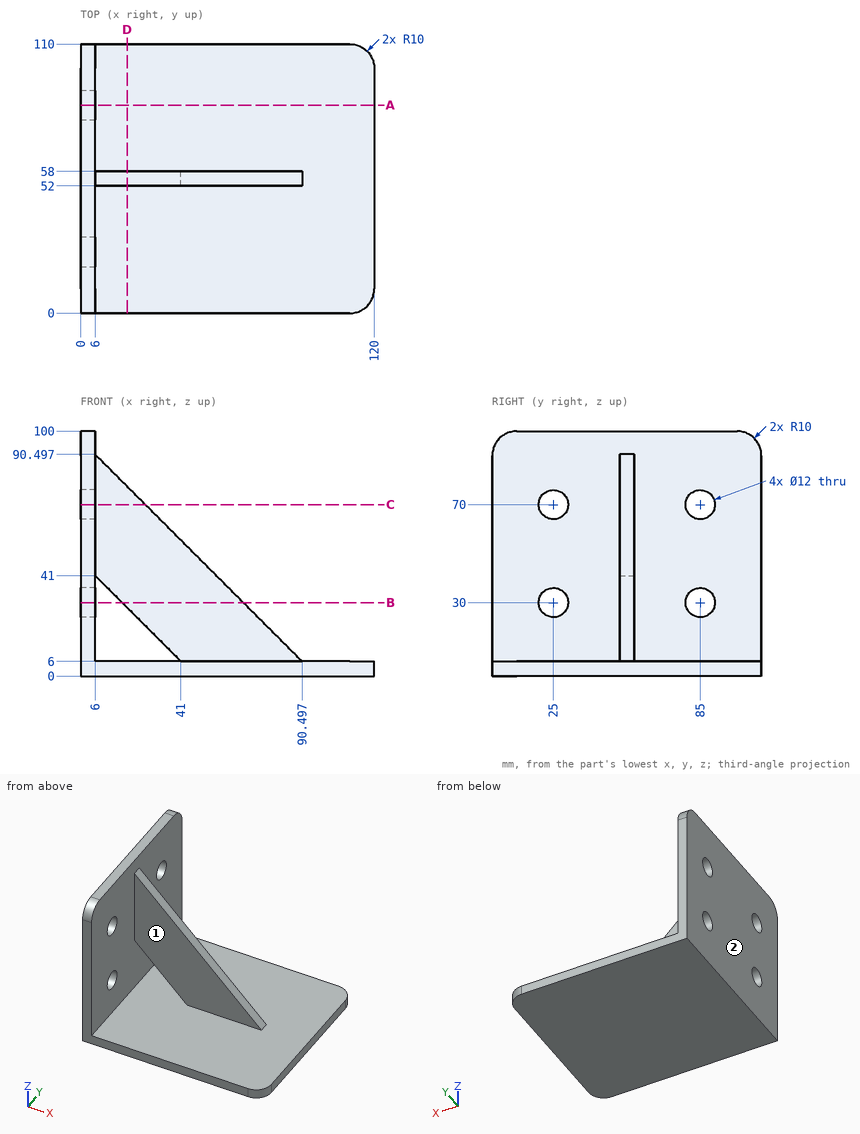
Verification items for this drawing (mm, ordinates from the low corner). Coordinates: 2 decimals unless noted, no trailing zeros. Order: outer loops, then holes, each group sorted by start corner. A loop starts at its lowest first (then second) coordinate and runs counter-clockwise, first axis right, second up. Notation, with made-up numbers: (25, 16.5) - (34, 16.5) arc R19 cw to (34, 29.5) - close; hole circle Ø9 at (-10.75, 4.5). An arc over 180 degrees is marked (long way). Answer as a JSON object with one key per item and string values. Group by question number.
Item 1: Sectioned sample at C-C, the plane z = 70. Record the cut outline in (x, y).
Item 2: Sectioned sample at D-D, the plane x = 19. Record the cut outline in (y, z), and give its area (3 significant figures).
Item 3: Depth check by flat-ended pin: pin 1 Ø11 at (y, z) = (25, 30) entering from +X; pin 2 Ø1 at (x, y) = (93, 98) entering from +Z; pin 3 Ø12 at (x, z) = (17, 32.5) entering from +Y. Enter the tip coordinate at first touch or a pass-through.
Item 4: Sectioned sample at B-B, the plane z = 30. Record the cut outline in (x, y).
Item 5: Draft check along X on the marked faces 1 and 2. Enter one of: +X half, -X half, draft (parallel to the pull), parting line (faces both ways), or undercut.
Item 6: Sectioned sample at A-A, the plane y = 85. Record the cut outline in (x, z).
Item 7: Scan lines: probe 1 along Z at (x, y) = (2.95, 85); probe 2 along X at (y, z) = (67.5, 87.5); probe 3 along Y at (x, z) = (9, 57.5). Record each from-to range of solid material in increasing order.
Resolved:
{
 "1": {"outline": "(0, 0) - (6, 0) - (6, 19) - (0, 19) - close; (0, 31) - (6, 31) - (6, 52) - (26.5, 52) - (26.5, 58) - (6, 58) - (6, 79) - (0, 79) - close; (0, 91) - (6, 91) - (6, 110) - (0, 110) - close"},
 "2": {"outline": "(0, 0) - (110, 0) - (110, 6) - (0, 6) - close; (52, 28) - (58, 28) - (58, 77.5) - (52, 77.5) - close", "area": "957 mm^2"},
 "3": {"pin 1": "through", "pin 2": "z = 6", "pin 3": "y = 58"},
 "4": {"outline": "(0, 0) - (6, 0) - (6, 19) - (0, 19) - close; (0, 31) - (6, 31) - (6, 79) - (0, 79) - close; (0, 91) - (6, 91) - (6, 110) - (0, 110) - close; (17, 52) - (66.5, 52) - (66.5, 58) - (17, 58) - close"},
 "5": {"face 1": "draft", "face 2": "-X half"},
 "6": {"outline": "(0, 0) - (120, 0) - (120, 6) - (6, 6) - (6, 24) - (0, 24) - close; (0, 36) - (6, 36) - (6, 64) - (0, 64) - close; (0, 76) - (6, 76) - (6, 100) - (0, 100) - close"},
 "7": {"probe 1": "0 to 24, 36 to 64, 76 to 100", "probe 2": "0 to 6", "probe 3": "52 to 58"}
}
